```python
from build123d import *

# Parameters (mm, degrees)
SKETCH2_R                                      = 12.7
BOSS_EXTRUDE6_DEPTH                            = 40.64
SKETCH3_R                                      = 3.5
CUT_EXTRUDE1_DEPTH                             = 40.64
SKETCH4_R                                      = 1.778
CUT_EXTRUDE2_DEPTH                             = 6
BOSS_EXTRUDE8_DEPTH                            = 10
SKETCH8_W                                      = 25.185693912
SKETCH8_H                                      = 10
BOSS_EXTRUDE9_DEPTH                            = 7.284789049
BOSS_EXTRUDE10_DEPTH                           = 30.64
CSK_FOR_M3_FLAT_HEAD_MACHINE_SCREW1_AT_2_COUNT = 2
CSK_FOR_M3_FLAT_HEAD_MACHINE_SCREW1_AT_2_PITCH = 9.039543014
CSK_FOR_M3_FLAT_HEAD_MACHINE_SCREW1_AT_3_COUNT = 2
CSK_FOR_M3_FLAT_HEAD_MACHINE_SCREW1_AT_3_PITCH = 9.039543014


with BuildPart() as part:
    # Sketch2 → Boss-Extrude6 (new body)
    with BuildSketch(Plane(origin=(0, -2111.389926236, 0), x_dir=(1, 0, 0), z_dir=(0, 1, 0))):
        with Locations(Location((-53.693967541, 163.840329354, 0), (0, 0, 180))):
            Circle(SKETCH2_R)
    extrude(amount=BOSS_EXTRUDE6_DEPTH)

    # Sketch3 → Cut-Extrude1 (cut)
    with BuildSketch(Plane(origin=(0, -2070.749926236, 0), x_dir=(1, 0, 0), z_dir=(0, 1, 0))):
        with Locations(Location((-53.693967541, 163.840329354, 0), (0, 0, 270))):
            Circle(SKETCH3_R)
    extrude(amount=-CUT_EXTRUDE1_DEPTH, mode=Mode.SUBTRACT)

    # Sketch4 → Cut-Extrude2 (cut)
    with BuildSketch(Plane.XZ.offset(2111.389926236)):
        with Locations(Location((-61.942859512, -159.077829354, 0), (0, 0, 270))):
            Circle(SKETCH4_R)
        with Locations(Location((-53.693967541, -173.365329354, 0), (0, 0, 270))):
            Circle(SKETCH4_R)
        with Locations(Location((-45.44507557, -159.077829354, 0), (0, 0, 270))):
            Circle(SKETCH4_R)
    extrude(amount=-CUT_EXTRUDE2_DEPTH, mode=Mode.SUBTRACT)

    # Sketch7 → Boss-Extrude8 (add)
    with BuildSketch(Plane.XZ.offset(2111.389926236)):
        with BuildLine():
            Line((-40.993967541, -163.840329354), (-40.993967541, -182.634287878))
            Line((-40.993967541, -182.634287878), (-66.179661453, -182.634287878))
            Line((-66.179661453, -182.634287878), (-66.179661453, -166.163570095))
            ThreePointArc((-66.179661453, -166.163570095), (-52.527415502, -176.486639343), (-40.993967541, -163.840329354))
        make_face()
    extrude(amount=-BOSS_EXTRUDE8_DEPTH)

    # Sketch8 → Boss-Extrude9 (add)
    with BuildSketch(Plane(origin=(0, 0, -182.634287878), x_dir=(-1, 0, 0), z_dir=(0, 0, -1))):
        with Locations((53.586814497, -2106.389926236)):
            Rectangle(SKETCH8_W, SKETCH8_H)
    extrude(amount=BOSS_EXTRUDE9_DEPTH)

    # Sketch9 → Boss-Extrude10 (add)
    with BuildSketch(Plane(origin=(0, -2070.749926236, 0), x_dir=(1, 0, 0), z_dir=(0, 1, 0))):
        with BuildLine():
            Line((-66.179661453, 163.840329354), (-66.179661453, 189.919076927))
            Line((-66.179661453, 189.919076927), (-40.993967541, 189.919076927))
            Line((-40.993967541, 189.919076927), (-40.993967541, 163.840329354))
            ThreePointArc((-40.993967541, 163.840329354), (-53.586814497, 176.43317631), (-66.179661453, 163.840329354))
        make_face()
    extrude(amount=-BOSS_EXTRUDE10_DEPTH)

    # Sketch15 → CSK for M3 Flat Head Machine Screw1 (revolve, cut)
    with BuildSketch(Plane(origin=(-53.586814498, -2075.749926236, -189.919076927), x_dir=(0, 1, 0), z_dir=(1, 0, 0))):
        Polygon((0, 0), (0, 10), (1.7, 8.978536948), (1.7, 1.45), (3.15, 0), align=None)
    csk_for_m3_flat_head_machine_screw1 = revolve(axis=Axis((-53.586814498, -2075.749926236, -196.269076927), (0, 0, 1)), mode=Mode.SUBTRACT)

    # CSK for M3 Flat Head Machine Screw1 at 2: CSK for M3 Flat Head Machine Screw1 ×2
    with Locations(*[(-i * CSK_FOR_M3_FLAT_HEAD_MACHINE_SCREW1_AT_2_PITCH, 0, 0) for i in range(1, CSK_FOR_M3_FLAT_HEAD_MACHINE_SCREW1_AT_2_COUNT)]):
        add(csk_for_m3_flat_head_machine_screw1, mode=Mode.SUBTRACT)

    # CSK for M3 Flat Head Machine Screw1 at 3: CSK for M3 Flat Head Machine Screw1 ×2
    with Locations(*[(i * CSK_FOR_M3_FLAT_HEAD_MACHINE_SCREW1_AT_3_PITCH, 0, 0) for i in range(1, CSK_FOR_M3_FLAT_HEAD_MACHINE_SCREW1_AT_3_COUNT)]):
        add(csk_for_m3_flat_head_machine_screw1, mode=Mode.SUBTRACT)

    # Mirror1: CSK for M3 Flat Head Machine Screw1 across plane
    add(csk_for_m3_flat_head_machine_screw1.mirror(Plane.ZX.offset(-2091.069926234)), mode=Mode.SUBTRACT)

    # Mirror1 copy 1 sketch → Mirror1 copy 1 (revolve, cut)
    with BuildSketch(Plane(origin=(-62.626357512, -2106.389926232, -189.919076927), x_dir=(0, -1, 0), z_dir=(1, 0, 0))):
        Polygon((0, 0), (0, -10), (1.7, -8.978536948), (1.7, -1.45), (3.15, 0), align=None)
    revolve(axis=Axis((-62.626357512, -2106.389926232, -196.269076927), (0, 0, -1)), mode=Mode.SUBTRACT)

    # Mirror1 copy 2 sketch → Mirror1 copy 2 (revolve, cut)
    with BuildSketch(Plane(origin=(-44.547271484, -2106.389926232, -189.919076927), x_dir=(0, -1, 0), z_dir=(1, 0, 0))):
        Polygon((0, 0), (0, -10), (1.7, -8.978536948), (1.7, -1.45), (3.15, 0), align=None)
    revolve(axis=Axis((-44.547271484, -2106.389926232, -196.269076927), (0, 0, -1)), mode=Mode.SUBTRACT)


solid = part.part
```
Design review of the part built by this model. Coordinates are the model's own, in mm. A direction names the side the tool comes from. Coordinates: 2 decimals unless noted, no trailing zeros. Loops run counter-clockwise (first coordinate to the right, second up) from the corner with the lowest first, then second, coordinate; pieces in that order, holes last. Notation, with made-up numbers: M 31,55 L 43,55 A36 cw 43,91 Z; hole C 12,-26.75 d9. An arc over 180 degrees is marked long. One line per question, with ' | ' between items.
(1) We need section B-B (y = -2085). Give the boundary of the cut face in (x, z).
Filled in:
outline: M -66.18,-189.92 L -40.99,-189.92 L -40.99,-163.84 A12.7 ccw long -66.18,-166.16 Z; hole C -53.69,-163.84 d7
(2) We need section A-A (z = -183.5). Give the boundary of the cut face in (x, y).
Filled in:
outline: M -66.18,-2111.39 L -40.99,-2111.39 L -40.99,-2070.75 L -66.18,-2070.75 Z; hole C -62.63,-2106.39 d3.4; hole C -62.63,-2075.75 d3.4; hole C -53.59,-2106.39 d3.4; hole C -53.59,-2075.75 d3.4; hole C -44.55,-2106.39 d3.4; hole C -44.55,-2075.75 d3.4
(3) We need section D-D (x = -48.5). Give the boundary of the cut face in (y, z), and give its area (3 significant figures).
Filled in:
outline: M -2111.39,-189.92 L -2070.75,-189.92 L -2070.75,-152.25 L -2111.39,-152.25 Z | area: 1,530 mm^2
(4) For pin 1 Ø2 at (x, y) = (-44.55, -2106.39) entering from +Z; pin 2 Ø1.5 at (y, z) = (-2083, -170) entering from -X; pin 3 Ø6 at (x, z) = (-52, -162.5) entering from +Y; pin 4 Ø4.5 at (x, y) = (-62.63, -2106.39) entering from -Z, all flat-tipped, find the tip position at first contact; note any pin that passes through.
Filled in:
pin 1: stops at z = -154.1 | pin 2: stops at x = -66.18 | pin 3: stops at y = -2070.75 | pin 4: stops at z = -189.02
(5) Draft analysis for pull direction X (two halves, no side actions). For faces 4 (the face through (-55.155, -2091.354, -151.225)), 5 (the face through (-51.93, -2108.43, -173.13)), 6 (the face through (-54, -2091, -189.919)), state which applies: released by +X, released by -X, zero draft, split by the parting line, or undercut.
Filled in:
face 4: split by the parting line | face 5: undercut | face 6: zero draft
(6) Wall thickness on probe 1 along Y at (x, z) = (-43.5, -187); probe 2 along Y at (x, z) = (-54, -187.5); probe 3 along X at (y, z) = (-2109.5, -186): over which ranges is each line inside the solid? List them lowest first.
Filled in:
probe 1: y = -2111.39 to -2107.73, -2105.05 to -2077.09, -2074.41 to -2070.75 | probe 2: y = -2111.39 to -2108.04, -2104.74 to -2077.4, -2074.1 to -2070.75 | probe 3: x = -66.18 to -40.99
(7) We need section C-C (z = -159.5). Give the boundary of the cut face in (x, y).
Filled in:
outline: M -65.63,-2111.39 L -63.67,-2111.39 L -63.67,-2105.39 L -60.22,-2105.39 L -60.22,-2111.39 L -47.17,-2111.39 L -47.17,-2105.39 L -43.72,-2105.39 L -43.72,-2111.39 L -41.76,-2111.39 L -41.76,-2070.75 L -65.63,-2070.75 Z
(8) Machinability: for faces 1 (the face through (-44.24, -2108.43, -157.77)), 2 (the face through (-44.62, -2077.45, -184.76)), 3 (the face through (-54, -2111.39, -170)), which of the approach directions +Z, -Z, +X, -X, +Y, -Y give a long, thin tool a straight path to every point of the face, cutting with its end or side? Answer none if there is none.
Filled in:
face 1: -Y | face 2: -Z | face 3: +Z, -Z, +X, -X, -Y
